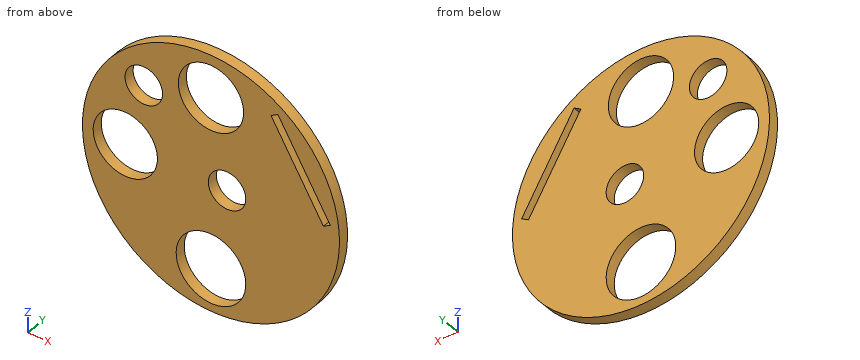
```python
from build123d import *

# Parameters (mm, degrees)
ESQUISSE1_R        = 24
ESQUISSE1_R_2      = 6.5
ESQUISSE1_R_3      = 6
ESQUISSE1_R_4      = 6.1
ESQUISSE1_R_5      = 3.5
BOSS_EXTRU_1_DEPTH = 2


with BuildPart() as part:
    # Esquisse1 → Boss.-Extru.1 (new body)
    with BuildSketch(Plane(origin=(0, 0, 0), x_dir=(1, 0, 0), z_dir=(0, 1, 0))):
        with Locations(Location((0, 0, 0), (0, 0, 270))):
            Circle(ESQUISSE1_R)
        with Locations(Location((0, 16, 0), (0, 0, 270))):
            Circle(ESQUISSE1_R_2, mode=Mode.SUBTRACT)
        with Locations(Location((-16, 0, 0), (0, 0, 270))):
            Circle(ESQUISSE1_R_3, mode=Mode.SUBTRACT)
        with Locations(Location((0, -16, 0), (0, 0, 270))):
            Circle(ESQUISSE1_R_4, mode=Mode.SUBTRACT)
        with Locations(Location((-12.542919229, -12.586407821, 0), (0, 0, 270))):
            Circle(ESQUISSE1_R_5, mode=Mode.SUBTRACT)
        with Locations(Location((3, 0, 0), (0, 0, 270))):
            Circle(ESQUISSE1_R_5, mode=Mode.SUBTRACT)
        Polygon((21, -1.535055726), (11.214276577, -17.821234439), (12.500027528, -18.593791552), (22.285750951, -2.307612838), align=None, mode=Mode.SUBTRACT)
    extrude(amount=BOSS_EXTRU_1_DEPTH)


solid = part.part
```
Part model, mm, in its own coordinate system. Round coordinates to 2 decimals unless told otherwise and drop trailing zeros. Write each loop counter-clockwise with the first axis right and the second up, starting at its lowest first coordinate (ties: lowest second). Pieces come first, ordered by that corner, then holes.
Item 1: Drop flat-ended pins along their axis: pin 1 Ø12 at (x, z) = (-17, -5.5) entering from -Y; pin 2 Ø6.5 at (x, z) = (-12.54, 12.59) entering from -Y. Give the stop position or say it passes through.
Results:
pin 1: stops at y = 0
pin 2: passes through
Item 2: Cut at A-A, the plane z = 15.5. Give the cut face in (x, y), plus the area to 3 significant figures.
Results:
outline: (-18.32, 0) - (-14.48, 0) - (-14.48, 2) - (-18.32, 2) - close; (-10.6, 0) - (-6.08, 0) - (-6.08, 2) - (-10.6, 2) - close; (6.08, 0) - (12.61, 0) - (12.61, 2) - (6.08, 2) - close; (14.36, 0) - (18.32, 0) - (18.32, 2) - (14.36, 2) - close
area: 37.7 mm2
Item 3: Cut at D-D, the plane x = 3. Give the cut face in (y, z).
Results:
outline: (0, -23.81) - (2, -23.81) - (2, -21.77) - (0, -21.77) - close; (0, -10.23) - (2, -10.23) - (2, -3.5) - (0, -3.5) - close; (0, 3.5) - (2, 3.5) - (2, 10.69) - (0, 10.69) - close; (0, 21.31) - (2, 21.31) - (2, 23.81) - (0, 23.81) - close
Item 4: Cut at C-C, the plane y = 1.4. Give the cut face in (x, z).
Results:
outline: circle Ø48 at (0, 0); hole circle Ø12 at (-16, 0); hole circle Ø7 at (-12.54, 12.59); hole circle Ø13 at (0, -16); hole circle Ø12.2 at (0, 16); hole circle Ø7 at (3, 0); hole (11.21, 17.82) - (21, 1.54) - (22.29, 2.31) - (12.5, 18.59) - close
Item 5: Cut at B-B, the plane x = -21. Give the cut face in (y, z).
Results:
outline: (0, -11.62) - (2, -11.62) - (2, -3.32) - (0, -3.32) - close; (0, 3.32) - (2, 3.32) - (2, 11.62) - (0, 11.62) - close
Item 6: Probe L1, parallel to X at y = 1.15, z = 0; L2, parallel to Z at x = 0.5, y = 1.85; L3, parallel to Z at x = -13, y = 0.7. List the from-to ranges inside material, lowest first.
Results:
L1: x = -24 to -22, -10 to -0.5, 6.5 to 24
L2: z = -23.99 to -22.48, -9.52 to -2.45, 2.45 to 9.92, 22.08 to 23.99
L3: z = -20.17 to -5.2, 5.2 to 9.12, 16.06 to 20.17
